from build123d import *

# Parameters (mm, degrees)
SKETCH1_W           = 57.667844522
SKETCH1_H           = 30
BOSS_EXTRUDE1_DEPTH = 30
SKETCH2_R           = 6
CUT_EXTRUDE2_DEPTH  = 40
CUT_EXTRUDE3_DEPTH  = 31
SKETCH8_R           = 1
CUT_EXTRUDE6_DEPTH  = 10
SKETCH10_R          = 3
CUT_EXTRUDE8_DEPTH  = 10


with BuildPart() as part:
    # Sketch1 → Boss-Extrude1 (new body)
    with BuildSketch(Plane(origin=(0, 0, 0), x_dir=(1, 0, 0), z_dir=(0, 1, 0))):
        Rectangle(SKETCH1_W, SKETCH1_H)
    extrude(amount=BOSS_EXTRUDE1_DEPTH)

    # Sketch2 → Cut-Extrude2 (cut)
    with BuildSketch(Plane(origin=(0, 30, 0), x_dir=(1, 0, 0), z_dir=(0, 1, 0))):
        with Locations((0, 4)):
            Circle(SKETCH2_R)
    extrude(amount=-CUT_EXTRUDE2_DEPTH, mode=Mode.SUBTRACT)

    # Sketch4 → Cut-Extrude3 (cut, through all)
    with BuildSketch(Plane(origin=(0, 30, 0), x_dir=(1, 0, 0), z_dir=(0, 1, 0))):
        with BuildLine():
            ThreePointArc((-4.5e-08, 15), (7.778174577, 11.778174609), (11, 4))
            Line((11, 4), (11, -12))
            Line((11, -12), (28.833922261, -12))
            Line((28.833922261, -12), (28.833922261, 15))
            Line((28.833922261, 15), (-4.5e-08, 15))
        make_face()
        with BuildLine():
            ThreePointArc((-11, 4), (-7.778174609, 11.778174577), (-4.5e-08, 15))
            Line((-4.5e-08, 15), (-28.833922261, 15))
            Line((-28.833922261, 15), (-28.833922261, -12))
            Line((-28.833922261, -12), (-11, -12))
            Line((-11, -12), (-11, 4))
        make_face()
    extrude(amount=-CUT_EXTRUDE3_DEPTH, mode=Mode.SUBTRACT)

    # Sketch8 → Cut-Extrude6 (cut)
    with BuildSketch(Plane(origin=(0, 30, 0), x_dir=(1, 0, 0), z_dir=(0, 1, 0))):
        with Locations((-8, 4)):
            Circle(SKETCH8_R)
        with Locations((8, 4)):
            Circle(SKETCH8_R)
    extrude(amount=-CUT_EXTRUDE6_DEPTH, mode=Mode.SUBTRACT)

    # Sketch10 → Cut-Extrude8 (cut)
    with BuildSketch(Plane(origin=(0, 0, 12), x_dir=(-1, 0, 0), z_dir=(0, 0, -1))):
        with Locations((19.916961131, 9)):
            Circle(SKETCH10_R)
        with Locations((-19.916961131, 9)):
            Circle(SKETCH10_R)
    extrude(amount=-CUT_EXTRUDE8_DEPTH, mode=Mode.SUBTRACT)


solid = part.part
Input: part model. Units: mm. Frame: model coordinates. A direction names the side the tool comes from. Give positions to 0.01 mm unless a question says otherwise; leave off trailing zeros. Order: outer loops, then holes, each group sorted by start corner. A loop starts at its lowest first (then second) coordinate and runs counter-clockwise, first axis right, second up.
Q1. Set-up query: faces 1 (the cylindrical face through (7.263, 25.07, -4.676)), 2 (the flat face through (-20, 15, 12)), 3 (the flat face through (20, 15, 12)). Return all of +Z, -Z, +X, -X, +Y, -Y with unobstructed straight access to the full face (end or side cutting, diameter ignored); none if empty.
Checked values:
face 1: +Y
face 2: -Z, -X, +Y, -Y
face 3: -Z, +X, +Y, -Y
Q2. Contact query for flat-ended pins moving along their axis: pin 1 Ø2.5 at (x, z) = (-8, -4) entering from -Y; pin 2 Ø10 at (x, y) = (13.5, 12.5) entering from -Z; pin 3 Ø14.5 at (x, y) = (24.5, 10) entering from -Z; pin 4 Ø8 at (y, z) = (15.5, 5.5) entering from -X. Output: stop coordinate, or through.
Checked values:
pin 1: stops at y = 0
pin 2: stops at z = -10.98
pin 3: stops at z = 12
pin 4: stops at x = -11
Q3. Section C-C on x = -19.5. Output: boundary loops of the cut face in (y, z), and give its area (3 significant figures).
Checked values:
outline: (0, 12) - (6.03, 12) - (6.03, 15) - (0, 15) - close; (11.97, 12) - (30, 12) - (30, 15) - (11.97, 15) - close
area: 72.2 mm2
Q4. Section B-B on y = 2.25. Output: boundary loops of the cut face in (x, z), and give its area (3 significant figures).
Checked values:
outline: (-28.83, 12) - (-11, 12) - (-11, -4) arc R11 ccw to (11, -4) - (11, 12) - (28.83, 12) - (28.83, 15) - (-28.83, 15) - close; hole circle Ø12 at (0, -4)
area: 602 mm2
Q5. Ray query, probe 1 along X at (y, z) = (23, -4); probe 2 along X at (y, z) = (14.5, -4); probe 3 along Z at (x, y) = (0, 21.25). Return the intervals inside material, ascending.
Checked values:
probe 1: x = -11 to -9, -7 to -6, 6 to 7, 9 to 11
probe 2: x = -11 to -6, 6 to 11
probe 3: z = -15 to -10, 2 to 15
Q6. Draft query along X for faces 4 (the flat face through (0, 30, 4)), 5 (the cylindrical face through (17.146, 7.851, 13.479)), 6 (the flat face through (11, 15, 4)), 7 (the flat face through (-8, 20, -4)). Return one class per face: +X half, -X half, draft (parallel to the pull), parting line (faces both ways), or undercut.
Checked values:
face 4: draft
face 5: undercut
face 6: +X half
face 7: undercut
Q7. Section A-A on y = 9. Output: boundary loops of the cut face in (x, z), and give its area (3 significant figures).
Checked values:
outline: (-28.83, 12) - (-22.92, 12) - (-22.92, 15) - (-28.83, 15) - close; (-16.92, 12) - (-11, 12) - (-11, -4) arc R11 ccw to (11, -4) - (11, 12) - (16.92, 12) - (16.92, 15) - (-16.92, 15) - close; (22.92, 12) - (28.83, 12) - (28.83, 15) - (22.92, 15) - close; hole circle Ø12 at (0, -4)
area: 566 mm2
Q8. Section D-D on z = -9. Output: boundary loops of the cut face in (x, y).
Checked values:
outline: (-9.8, 0) - (-3.32, 0) - (-3.32, 30) - (-9.8, 30) - close; (3.32, 0) - (9.8, 0) - (9.8, 30) - (3.32, 30) - close
